from build123d import *

# Parameters (mm, degrees)
SKETCH3_R           = 22.225
SKETCH3_R_2         = 2.778125
SKETCH3_W           = 3.175
SKETCH3_H           = 6.35
BOSS_EXTRUDE1_DEPTH = 3.175


with BuildPart() as part:
    # Sketch3 → Boss-Extrude1 (new body)
    with BuildSketch(Plane(origin=(0, 0, 0), x_dir=(1, 0, 0), z_dir=(0, 1, 0))):
        with BuildLine():
            Line((0, 0), (0, 114.3))
            ThreePointArc((0, 114.3), (0.796571799, 123.260868714), (3.161305831, 131.940714778))
            Line((3.161305831, 131.940714778), (42.852914082, 239.127776658))
            ThreePointArc((42.852914082, 239.127776658), (76.2, 262.339276313), (109.547085918, 239.127776658))
            Line((109.547085918, 239.127776658), (149.238694169, 131.940714778))
            ThreePointArc((149.238694169, 131.940714778), (151.603428201, 123.260868714), (152.4, 114.3))
            Line((152.4, 114.3), (152.4, 0))
            Line((152.4, 0), (0, 0))
        make_face()
        with Locations(Location((76.2, 184.24413735, 0), (0, 0, 270))):
            Circle(SKETCH3_R, mode=Mode.SUBTRACT)
        with Locations(Location((103.98125, 184.24413735, 0), (0, 0, 270))):
            Circle(SKETCH3_R_2, mode=Mode.SUBTRACT)
        with Locations(Location((48.41875, 184.24413735, 0), (0, 0, 90))):
            Circle(SKETCH3_R_2, mode=Mode.SUBTRACT)
        with Locations((20.0285604, 13.212735966)):
            Rectangle(SKETCH3_W, SKETCH3_H, mode=Mode.SUBTRACT)
        with Locations((132.3714396, 13.212735966)):
            Rectangle(SKETCH3_W, SKETCH3_H, mode=Mode.SUBTRACT)
    extrude(amount=BOSS_EXTRUDE1_DEPTH)


solid = part.part
Geometry check sheet. Reference: the model listing, model coordinates, mm. Round coordinates to 2 decimals unless told otherwise and drop trailing zeros. Write each loop counter-clockwise with the first axis right and the second up, starting at its lowest first coordinate (ties: lowest second). Pieces come first, ordered by that corner, then holes. Notation, with made-up numbers: (-3.75, -6.5) -> (33.25, -6.5) arc R21 cw to (33.25, 27.5) -> close; hole circle Ø4 at (-13.5, -15.75). An arc over 180 degrees is marked (long way). One line per item, written item: value. Start each with the question number.
(1) Cross-section at A-A, the plane x = 76.2. Record the cut outline in (y, z) (3 decimals), and give its area (3 significant figures).
(2) Go/stop test with a flat-tipped pin: pin 1 Ø4.5 at (x, z) = (48.42, -184.24) entering from -Y. Record where the tip stops, or that it passes through.
(3) Cross-section at B-B, the plane y = 1.6. Record the cut outline in (x, z) (3 decimals), and give its area (3 significant figures).
(4) Draft check along Z on faces 1 (the flat face through (22.729, 1.565, -184.784)), 2 (the flat face through (77, 0, -104)), 3 (the cylindrical face through (48.3, 1.57, -181.47)), 4 (the cylindrical face through (62.7, 1.6, -201.9)). Enter one of: +Z half, -Z half, draft (parallel to the pull), parting line (faces both ways), or undercut.
(5) Cross-section at C-C, the plane z = -173. Record the cut outline in (x, y) (3 decimals).
(6) Scan lines: line 1 (Z direction, x = 94.5, y = 1.8); line 2 (Z direction, x = 65.5, y = 0.65); line 3 (X direction, y = 1.65, z = -204). Record each from-to range of solid material in increasing order. Write a range as [from, to].
Answer:
1. outline: (0, -262.339) -> (3.175, -262.339) -> (3.175, -206.469) -> (0, -206.469) -> close; (0, -162.019) -> (3.175, -162.019) -> (3.175, 0) -> (0, 0) -> close
1. area: 692 mm²
2. pin 1: through
3. outline: (0, -114.3) arc R50.8 ccw to (3.161, -131.941) -> (42.853, -239.128) arc R35.56 ccw to (109.547, -239.128) -> (149.239, -131.941) arc R50.8 ccw to (152.4, -114.3) -> (152.4, 0) -> (0, 0) -> close; hole (18.441, -16.388) -> (21.616, -16.388) -> (21.616, -10.038) -> (18.441, -10.038) -> close; hole circle Ø5.556 at (48.419, -184.244); hole circle Ø44.45 at (76.2, -184.244); hole circle Ø5.556 at (103.981, -184.244); hole (130.784, -16.388) -> (133.959, -16.388) -> (133.959, -10.038) -> (130.784, -10.038) -> close
3. area: 31,000 mm²
4. face 1: -Z half
4. face 2: draft
4. face 3: undercut
4. face 4: undercut
5. outline: (18.366, 0) -> (57.029, 0) -> (57.029, 3.175) -> (18.366, 3.175) -> close; (95.371, 0) -> (134.034, 0) -> (134.034, 3.175) -> (95.371, 3.175) -> close
6. line 1: [-257.27, -196.86], [-171.63, 0]
6. line 2: [-260.69, -203.72], [-164.76, 0]
6. line 3: [29.85, 66.02], [86.38, 122.55]
